from build123d import *

# Parameters (mm, degrees)
SKETCH_1_R          = 1.525
EXTRUDE_1_DEPTH     = 6
SKETCH_4_W          = 2.5
SKETCH_4_H          = 105.086243491
EXTRUDE_3_DEPTH     = 85
CUT_EXTRUDE_1_DEPTH = 58
SKETCH_5_W          = 85.517137539
SKETCH_5_H          = 212
CUT_EXTRUDE_2_DEPTH = 4


with BuildPart() as part:
    # 草图1 → 凸台-拉伸1 (new body)
    with BuildSketch(Plane(origin=(0, 0, 0), x_dir=(1, 0, 0), z_dir=(0, 1, 0))):
        Polygon((0, 200.086243491), (70.15383623, 200.086243491), (70.15383623, 107.080558208), (70.15383623, -11.913756509), (-28.642514872, -11.913756509), (-28.642514872, 0.086243491), (-28.642514872, 200.086243491), (-10.033645843, 200.086243491), align=None)
        with Locations(Location((-24.222040848, 145, 0), (0, 0, 270))):
            Circle(SKETCH_1_R, mode=Mode.SUBTRACT)
        with Locations(Location((66.977959152, 145, 0), (0, 0, 270))):
            Circle(SKETCH_1_R, mode=Mode.SUBTRACT)
        with Locations(Location((66.977959152, 35, 0), (0, 0, 270))):
            Circle(SKETCH_1_R, mode=Mode.SUBTRACT)
        with Locations(Location((-24.222040848, 35, 0), (0, 0, 270))):
            Circle(SKETCH_1_R, mode=Mode.SUBTRACT)
        with Locations(Location((-24.222040848, 10.701543846, 0), (0, 0, 270))):
            Circle(SKETCH_1_R, mode=Mode.SUBTRACT)
        with Locations(Location((66.977959152, 10.701543846, 0), (0, 0, 270))):
            Circle(SKETCH_1_R, mode=Mode.SUBTRACT)
        with Locations(Location((66.977959152, 168.701543846, 0), (0, 0, 270))):
            Circle(SKETCH_1_R, mode=Mode.SUBTRACT)
        with Locations(Location((-24.222040848, 168.701543846, 0), (0, 0, 270))):
            Circle(SKETCH_1_R, mode=Mode.SUBTRACT)
        with BuildLine():
            Line((61.212367219, -4.489544392), (6.977959152, -4.489544392))
            ThreePointArc((6.977959152, -4.489544392), (4.977959152, -2.489544392), (6.977959152, -0.489544392))
            Line((6.977959152, -0.489544392), (8.977959152, -0.489544392))
            Line((8.977959152, -0.489544392), (28.977959152, -0.489544392))
            Line((28.977959152, -0.489544392), (32.977959152, -0.489544392))
            Line((32.977959152, -0.489544392), (52.977959152, -0.489544392))
            Line((52.977959152, -0.489544392), (56.977959152, -0.489544392))
            Line((56.977959152, -0.489544392), (61.212367219, -0.489544392))
            ThreePointArc((61.212367219, -0.489544392), (63.212367219, -2.489544392), (61.212367219, -4.489544392))
        make_face(mode=Mode.SUBTRACT)
        with BuildLine():
            Line((8.977959152, 109.497464931), (8.977959152, 61.518458116))
            ThreePointArc((8.977959152, 61.518458116), (6.977959152, 59.518458116), (4.977959152, 61.518458116))
            Line((4.977959152, 61.518458116), (4.977959152, 109.497464931))
            ThreePointArc((4.977959152, 109.497464931), (6.977959152, 111.497464931), (8.977959152, 109.497464931))
        make_face(mode=Mode.SUBTRACT)
        with BuildLine():
            Line((4.977959152, 190.683676085), (4.977959152, 175.850262547))
            ThreePointArc((4.977959152, 175.850262547), (6.977959152, 173.850262547), (8.977959152, 175.850262547))
            Line((8.977959152, 175.850262547), (8.977959152, 190.683676085))
            ThreePointArc((8.977959152, 190.683676085), (6.977959152, 192.683676085), (4.977959152, 190.683676085))
        make_face(mode=Mode.SUBTRACT)
        with BuildLine():
            Line((32.977959152, 190.683676085), (32.977959152, 174.729552713))
            ThreePointArc((32.977959152, 174.729552713), (30.977959152, 172.729552713), (28.977959152, 174.729552713))
            Line((28.977959152, 174.729552713), (28.977959152, 190.683676085))
            ThreePointArc((28.977959152, 190.683676085), (30.977959152, 192.683676085), (32.977959152, 190.683676085))
        make_face(mode=Mode.SUBTRACT)
        with BuildLine():
            Line((56.977959152, 94.393526779), (56.977959152, 22.664710655))
            ThreePointArc((56.977959152, 22.664710655), (54.977959152, 20.664710655), (52.977959152, 22.664710655))
            Line((52.977959152, 22.664710655), (52.977959152, 94.393526779))
            ThreePointArc((52.977959152, 94.393526779), (54.977959152, 96.393526779), (56.977959152, 94.393526779))
        make_face(mode=Mode.SUBTRACT)
        with BuildLine():
            Line((28.977959152, 109.497464931), (28.977959152, 22.664710655))
            ThreePointArc((28.977959152, 22.664710655), (30.977959152, 20.664710655), (32.977959152, 22.664710655))
            Line((32.977959152, 22.664710655), (32.977959152, 109.497464931))
            ThreePointArc((32.977959152, 109.497464931), (30.977959152, 111.497464931), (28.977959152, 109.497464931))
        make_face(mode=Mode.SUBTRACT)
    extrude(amount=EXTRUDE_1_DEPTH)

    # 草图4 → 凸台-拉伸3 (add)
    with BuildSketch(Plane.XZ):
        with Locations((-29.892514872, -147.543121746)):
            Rectangle(SKETCH_4_W, SKETCH_4_H)
    extrude(amount=-EXTRUDE_3_DEPTH)

    # 草图3 → 切除-拉伸1 (cut)
    with BuildSketch(Plane(origin=(-28.642514872, 0, 0), x_dir=(0, 0, -1), z_dir=(1, 0, 0))):
        with BuildLine():
            Line((113.273012401, 18), (113.273012401, 67.892967917))
            ThreePointArc((113.273012401, 67.892967917), (115.023012401, 69.642967917), (116.773012401, 67.892967917))
            Line((116.773012401, 67.892967917), (116.773012401, 18))
            ThreePointArc((116.773012401, 18), (115.023012401, 16.25), (113.273012401, 18))
        make_face()
        with BuildLine():
            Line((180.773012401, 18), (180.773012401, 67.892967917))
            ThreePointArc((180.773012401, 67.892967917), (179.023012401, 69.642967917), (177.273012401, 67.892967917))
            Line((177.273012401, 67.892967917), (177.273012401, 18))
            ThreePointArc((177.273012401, 18), (179.023012401, 16.25), (180.773012401, 18))
        make_face()
    extrude(amount=-CUT_EXTRUDE_1_DEPTH, mode=Mode.SUBTRACT)

    # 草图5 → 切除-拉伸2 (cut)
    with BuildSketch(Plane.XZ):
        with Locations((21.659274281, -94.086243491)):
            Rectangle(SKETCH_5_W, SKETCH_5_H)
    extrude(amount=-CUT_EXTRUDE_2_DEPTH, mode=Mode.SUBTRACT)


solid = part.part
Source: CAD feature listing. Evaluate the final solid. Frame: model axes, mm. A direction names the side the tool comes from. Coordinates: 2 decimals unless noted, no trailing zeros. Loops run counter-clockwise (first coordinate to the right, second up) from the corner with the lowest first, then second, coordinate; pieces in that order, holes last. Notation, with made-up numbers: (76.5, 86.25) - (122.5, 86.25) arc R12 cw to (122.5, 91.25) - close; hole circle Ø11 at (14, 3.25). An arc over 180 degrees is marked (long way). Return JSON: item names as keys, results as strings.
Q1. Material intervals for line 1 along X through (y, z) = (3, -35); line 2 along Y through (x, z) = (60, -172); line 3 along X through (y, z) = (76, -115), sorted ascending.
Results:
{"line 1": "-28.64 to -25.75, -22.7 to -21.1, 64.42 to 65.45, 68.5 to 70.15", "line 2": "4 to 6", "line 3": "-31.14 to -28.64"}
Q2. Section D-D, the plane y = 10. Return loops of the section in (x, z).
Results:
{"outline": "(-31.14, -200.09) - (-28.64, -200.09) - (-28.64, -95) - (-31.14, -95) - close"}
Q3. Section A-A, the plane z = -47.5. Return loops of the section in (x, y), plus the area to 3 significant figures.
Results:
{"outline": "(-28.64, 0) - (-21.1, 0) - (-21.1, 4) - (28.98, 4) - (28.98, 6) - (-28.64, 6) - close; (32.98, 4) - (52.98, 4) - (52.98, 6) - (32.98, 6) - close; (56.98, 4) - (64.42, 4) - (64.42, 0) - (70.15, 0) - (70.15, 6) - (56.98, 6) - close", "area": "235 mm2"}
Q4. Access query for faces 4 (the flat face through (-28.643, 45, -148)), 5 (the flat face through (21, 4, -93)), 6 (the flat face through (21.4, 4.3, 11.914)). Directions: +Z, -Z, +X, -X, +Y, -Y. A direction counts if a zero-diameter tool reaches every point of the face in a straight line with its end or side. Return the directions, or none.
Results:
{"face 4": "+Z, -Z, +X, +Y", "face 5": "+Z, -Z, -Y", "face 6": "+Z, +X, -X, +Y, -Y"}
Q5. Mould query, pull axis X, two halves, no side actions, for faces 1 (the flat face through (-28.643, 3, -42)), 2 (the flat face through (-26, 0, -93)), 3 (the flat face through (64.418, 2, -96)). Classes: released by +X, released by -X, zero draft, split by the parting line, or undercut.
Results:
{"face 1": "released by -X", "face 2": "zero draft", "face 3": "undercut"}
Q6. Section C-C, the plane x = 23. Return loops of the section in (y, z), plus the area to 3 significant figures.
Results:
{"outline": "(4, -200.09) - (6, -200.09) - (6, 0.49) - (4, 0.49) - close; (4, 4.49) - (6, 4.49) - (6, 11.91) - (4, 11.91) - close", "area": "416 mm2"}
Q7. Section B-B, the plane y = 53. Return loops of the section in (x, z), plus the area to 3 significant figures.
Results:
{"outline": "(-31.14, -200.09) - (-28.64, -200.09) - (-28.64, -180.77) - (-31.14, -180.77) - close; (-31.14, -177.27) - (-28.64, -177.27) - (-28.64, -116.77) - (-31.14, -116.77) - close; (-31.14, -113.27) - (-28.64, -113.27) - (-28.64, -95) - (-31.14, -95) - close", "area": "245 mm2"}
Q8. Contact query for flat-ended pins moving along their axis: P1, Ø5, axis at y = 4.5, z = -57.5, coming from the -X side; P2, Ø6, axis at x = 54.5, z = -94.5, coming from the +Y side; P3, Ø0.8, axis at x = -29.5, y = 50, coming from the +Z side; P4, Ø4, axis at x = -24.22, z = -35, coming from the -Y side. Output: stop coordinate, or through.
Results:
{"P1": "x = -28.64", "P2": "y = 6", "P3": "z = -95", "P4": "y = 0"}
